from build123d import *

# Parameters (mm, degrees)
F0_R     = 38.1
F1_DEPTH = 5.08
F3_DEPTH = 5.08
F4_R     = 4.679015
F5_DEPTH = 25.4


with BuildPart() as f1:
    # F0 (on Top) → F1 (new body)
    with BuildSketch(Plane.XY):
        Circle(F0_R)
    extrude(amount=-F1_DEPTH)

    # F2 (on Top) → F3 (join)
    with BuildSketch(Plane.XY):
        with BuildLine():
            ThreePointArc((6.714925, -4.061114), (7.559037, -2.108039), (7.847475, 0))
            ThreePointArc((7.847475, 0), (6.10013, 4.936729), (1.636232, 7.674999))
            ThreePointArc((1.636232, 7.674999), (-0.362003, 7.839121), (-2.336609, 7.491537))
            ThreePointArc((-2.336609, 7.491537), (-7.713703, 1.442794), (-4.88639, -6.140526))
            ThreePointArc((-4.88639, -6.140526), (-3.20497, -7.163173), (-1.321987, -7.735323))
            ThreePointArc((-1.321987, -7.735323), (0.937058, -7.791328), (3.118403, -7.20128))
            ThreePointArc((3.118403, -7.20128), (5.161274, -5.911356), (6.714925, -4.061114))
        make_face()
        with BuildLine():
            ThreePointArc((-2.336609, 7.491537), (-0.362003, 7.839121), (1.636232, 7.674999))
            add(Edge.make_bspline(
                [(4.922261, 37.561897), (-3.396095, 27.139671), (-3.426963, 16.903229), (1.636232, 7.674999)],
                knots=[0, 0, 0, 0, 30.067003, 30.067003, 30.067003, 30.067003], degree=3))
            Line((4.922261, 37.561897), (0, 37.607454))
            add(Edge.make_bspline(
                [(-2.336609, 7.491537), (-9.098259, 16.218371), (-10.203362, 26.240014), (0, 37.607454)],
                knots=[0, 0, 0, 0, 30.206426, 30.206426, 30.206426, 30.206426], degree=3))
        make_face()
        with BuildLine():
            add(Edge.make_bspline(
                [(6.714925, -4.061114), (20.714046, -4.037036), (23.886483, -5.73107), (31.794433, -20.356581)],
                knots=[0, 0, 0, 0, 29.908592, 29.908592, 29.908592, 29.908592], degree=3))
            ThreePointArc((6.714925, -4.061114), (5.161274, -5.911356), (3.118403, -7.20128))
            add(Edge.make_bspline(
                [(3.118403, -7.20128), (16.17207, -7.814267), (20.896574, -10.618221), (29.992331, -23.169141)],
                knots=[0, 0, 0, 0, 31.259888, 31.259888, 31.259888, 31.259888], degree=3))
            Line((29.992331, -23.169141), (31.794433, -20.356581))
        make_face()
        with BuildLine():
            ThreePointArc((-1.321987, -7.735323), (-3.20497, -7.163173), (-4.88639, -6.140526))
            add(Edge.make_bspline(
                [(-4.88639, -6.140526), (-6.197293, -16.774258), (-15.328656, -23.210278), (-26.230019, -27.077071)],
                knots=[0, 0, 0, 0, 29.897983, 29.897983, 29.897983, 29.897983], degree=3))
            Line((-26.230019, -27.077071), (-22.290342, -30.278141))
            add(Edge.make_bspline(
                [(-1.321987, -7.735323), (-1.265044, -20.887848), (-9.577676, -27.635643), (-22.290342, -30.278141)],
                knots=[0, 0, 0, 0, 30.787181, 30.787181, 30.787181, 30.787181], degree=3))
        make_face()
    extrude(amount=F3_DEPTH)

    # F4 (on face) → F5 (cut)
    with BuildSketch(Plane.XY.offset(5.08)):
        Circle(F4_R)
    extrude(amount=-F5_DEPTH, mode=Mode.SUBTRACT)


solid = f1.part
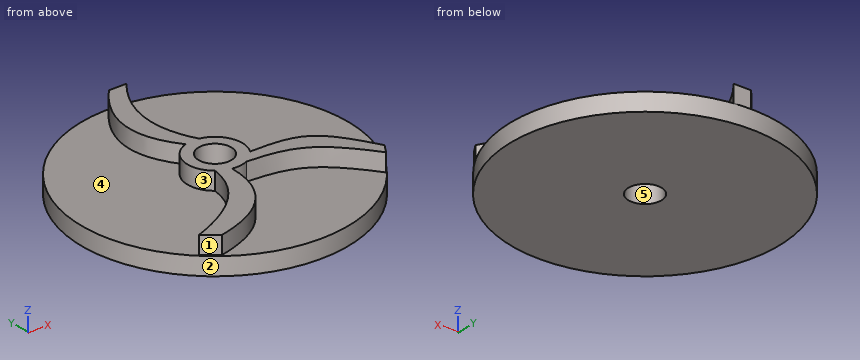
Could you check a few things on this model? Use its own coordinates, in mm. Face numbers are marked on the shaded views. A direction names the side the tool comes from. Coordinates: 2 decimals unless noted, no trailing zeros. Write each loop counter-clockwise with the first axis right and the second up, starting at its lowest first coordinate (ties: lowest second). Pieces come first, ordered by that corner, then holes. Notation, with made-up numbers: (56.25, 37) - (103.25, 37) arc R25 ccw to (103.25, 52) - close; hole circle Ø5 at (13.25, 28). An arc over 180 degrees is marked (long way). Put each result on its own line as item: value. Start each with the question number.
Q1. I'm going to push flat-ended pins straight in: P1, Ø8, axis at x = 25.5, y = -10, coming from the +Z side; P2, Ø5, axis at y = -26, z = -2.5, coming from the +X side; P3, Ø5, axis at x = 8, y = 17.5, coming from the +Z side; P4, Ø1, axis at y = -28, z = -1.5, coming from the +X side. Where does each tip first touch, or does it pass through?
Q2. I want a section at B-B on z = -4. Write out the boundary of the cut face in (x, y).
Q3. Thinking about a two-plate mould opening in Y: for the marked faces 1, 2 and 3, which applies, pulls with the +Y half, pulls with the -Y half, needs draft (parallel to the pull), parting line crosses it, or undercut?
Q4. I want a section at D-D on x = -33. Write out the boundary of the cut face in (y, z), plus the area to 3 significant figures.
Q5. Please list where these lines run through material, in increasing order: L1, parallel to Y at x = 0, z = -2.5; L2, parallel to Z at x = -21.5, y = 8; L3, parallel to Y at x = -4, z = -0.75.
Q6. I want a section at A-A on y = -3. Write out the boundary of the cut face in (x, z), plus the area to 3 significant figures.
Q7. Which directions (+Z, -Z, +X, -X, +Y, -Y) give clear straight access to the entire face, cutting with the end or side of a thin tool? Please do the marked faces 4 and 5.
Q8. I want a section at C-C on y = 6.5. Write out the boundary of the cut face in (x, z), plus the area to 3 significant figures.
Checks:
1. P1: z = 5.08
1. P2: x = 29.99
1. P3: z = 0
1. P4: x = 26.37
2. outline: circle Ø76.2 at (0, 0); hole circle Ø9.36 at (0, 0)
3. face 1: pulls with the -Y half
3. face 2: parting line crosses it
3. face 3: undercut
4. outline: (-19.04, -5.08) - (19.04, -5.08) - (19.04, 0) - (-19.04, 0) - close
4. area: 193 mm²
5. L1: -38.1 to -4.68, 4.68 to 38.1
5. L2: -5.08 to 0
5. L3: -37.89 to -2.43, 2.43 to 37.89
6. outline: (-37.98, -5.08) - (-3.59, -5.08) - (-3.59, 5.08) - (-7.25, 5.08) - (-7.25, 0) - (-37.98, 0) - close; (3.59, -5.08) - (37.98, -5.08) - (37.98, 0) - (7.25, 0) - (7.25, 5.08) - (3.59, 5.08) - close
6. area: 387 mm²
7. face 4: +Z
7. face 5: +Z, -Z
8. outline: (-37.54, -5.08) - (37.54, -5.08) - (37.54, 0) - (4.4, 0) - (4.4, 5.08) - (-4.4, 5.08) - (-4.4, 0) - (-37.54, 0) - close
8. area: 426 mm²
